```python
from build123d import *

# Parameters (mm, degrees)
F0_R     = 23.749
F1_DEPTH = 3.1242
F2_R     = 14.2875
F3_DEPTH = 7.1628


with BuildPart() as f1:
    # F0 (on Front) → F1 (new body)
    with BuildSketch(Plane.XZ):
        Circle(F0_R)
        with BuildLine():
            ThreePointArc((6.174591, -1.5875), (-6.3754, 0), (6.174591, 1.5875))
            Line((6.174591, 1.5875), (8.555841, 1.5875))
            Line((8.555841, 1.5875), (8.555841, -1.5875))
            Line((8.555841, -1.5875), (6.174591, -1.5875))
        make_face(mode=Mode.SUBTRACT)
    extrude(amount=F1_DEPTH)

    # F2 (on face) → F3 (join)
    with BuildSketch(Plane.XZ.offset(3.1242)):
        Circle(F2_R)
        with BuildLine():
            ThreePointArc((6.174591, -1.5875), (-6.3754, 0), (6.174591, 1.5875))
            Line((6.174591, 1.5875), (8.555841, 1.5875))
            Line((8.555841, 1.5875), (8.555841, -1.5875))
            Line((8.555841, -1.5875), (6.174591, -1.5875))
        make_face(mode=Mode.SUBTRACT)
    extrude(amount=F3_DEPTH)


solid = f1.part
```
Could you check a few things on this model? Use its own coordinates, in mm. A direction names the side the tool comes from. Give positions to 0.01 mm unless a question says otherwise; leave off trailing zeros. Order: outer loops, then holes, each group sorted by start corner. A loop starts at its lowest first (then second) coordinate and runs counter-clockwise, first axis right, second up.
Q1. I'm going to push flat-ended pins straight in: P1, Ø2, axis at x = -13, z = -18.5, coming from the -Y side; P2, Ø3.5, axis at y = -5.5, z = 1, coming from the -X side; P3, Ø1.5, axis at y = -5, z = -7, coming from the +X side. Where does each tip first touch, or does it pass through?
Q2. Suppose I cut it at A-A, the plane z = 0. Write out the boundary of the cut face in (x, y), and give its area (3 significant figures).
Q3. Suppose I cut it at D-D, the plane x = 12.5. Write out the boundary of the cut face in (y, z).
Q4. We'd pull the mould along X, two halves only. Please class faces 4 (the flat face through (5, 0, -5)), 5 (the cylindrical face through (-14.274, -6.655, 0.628)), 6 (the flat face through (8.556, -5, 0)), 7 (the cylindrical face through (-6.37, -5.07, -0.26)): +X half, -X half, draft (parallel to the pull), parting line (faces both ways), or undercut.
Q5. Suppose I cut it at C-C, the plane y = -0.75. Write out the boundary of the cut face in (x, z).
Q6. Suppose I cut it at B-B, the plane x = 0. Write out the boundary of the cut face in (y, z), and give its area (3 significant figures).
Q7. For faces 1 (the flat face through (7, -5, 1.588)), 2 (the flat face through (10.22, -3.124, -10.22)), 3 (the flat face through (6, -10.287, -3)), which set-ups out of +Z, -Z, +X, -X, +Y, -Y let a thin tool reach every point of the face, with its end or its side?
Q8. If I drill on line 1 along Z through (x, y) = (0, -7.75); line 2 along Y through (x, z) = (-4.5, -16.5); line 3 along Z through (x, y) = (-1, -1.75), over which ranges is the centre line in solid material (lowest first)?
Solution:
1. P1: stops at y = -3.12
1. P2: stops at x = -14.29
1. P3: stops at x = 12.85
2. outline: (-23.75, -3.12) - (-14.29, -3.12) - (-14.29, -10.29) - (-6.38, -10.29) - (-6.38, 0) - (-23.75, 0) - close; (8.56, -10.29) - (14.29, -10.29) - (14.29, -3.12) - (23.75, -3.12) - (23.75, 0) - (8.56, 0) - close
2. area: 199 mm2
3. outline: (-10.29, -6.92) - (-3.12, -6.92) - (-3.12, -20.19) - (0, -20.19) - (0, 20.19) - (-3.12, 20.19) - (-3.12, 6.92) - (-10.29, 6.92) - close
4. face 4: draft
4. face 5: parting line
4. face 6: undercut
4. face 7: undercut
5. outline: circle Ø47.5 at (0, 0); hole (6.17, -1.59) - (8.56, -1.59) - (8.56, 1.59) - (6.17, 1.59) arc R6.38 ccw (long way) to start
6. outline: (-10.29, -14.29) - (-3.12, -14.29) - (-3.12, -23.75) - (0, -23.75) - (0, -6.38) - (-10.29, -6.38) - close; (-10.29, 6.38) - (0, 6.38) - (0, 23.75) - (-3.12, 23.75) - (-3.12, 14.29) - (-10.29, 14.29) - close
6. area: 222 mm2
7. face 1: +Y, -Y
7. face 2: -Y
7. face 3: +Z, -Z, +X, -X, -Y
8. line 1: z = -14.29 to -6.38, 6.38 to 14.29
8. line 2: y = -3.12 to 0
8. line 3: z = -23.73 to -6.3, 6.3 to 23.73
